For this review, take the finished solid that the model builds, in its own axes (mm). A direction names the side the tool comes from. Coordinates: 2 decimals unless noted, no trailing zeros. Write each loop counter-clockwise with the first axis right and the second up, starting at its lowest first coordinate (ties: lowest second). Pieces come first, ordered by that corner, then holes. Notation, with made-up numbers: M -40,86.5 L 7,86.5 A23 cw 7,113.5 Z; hole C 37.5,66.5 d1. An arc over 180 degrees is marked long. One line per question, with ' | ' between items.
from build123d import *

# Parameters (mm, degrees)
F0_R         = 1
F0_W         = 18
F0_H         = 10
F1_DEPTH     = 5
F0_W_2       = 21.25
F0_R_2       = 4
F2_DEPTH     = 20
F3_R         = 4
F4_DEPTH     = 25
F5_DEPTH     = 5
F6_T4_DEPTH  = 18
F7_T1_DEPTH  = 5
F7_T3_DEPTH  = 18
F7_T8_DEPTH  = 10
F7_T13_DEPTH = 10
F7_T19_DEPTH = 22.8584149398
F7_T24_DEPTH = 17.8584149398
F7_T33_DEPTH = 30.8584149398
F7_S35_R     = 4
F7_T36_DEPTH = 17
F7_T39_DEPTH = 17.8584149398
F7_S41_R     = 4
F7_T42_DEPTH = 11
F7_T48_DEPTH = 30.8584149398
F7_S50_R     = 4
F7_T51_DEPTH = 17
F7_T54_DEPTH = 17.8584149398
F7_S56_R     = 4
F7_T57_DEPTH = 11
F7_T63_DEPTH = 17.8584149398
F7_T69_DEPTH = 22.8584149398


# Not quite as in the source:
# - a fillet or chamfer that OpenCascade refuses, or shapes differently, is made with other operations: its cross-section is extruded or revolved along the edge and cut away or added
# - a feature names something its author has since deleted; it is built from what else it names


with BuildPart() as f1:
    # F0 (on Top) → F1 (new body)
    with BuildSketch(Plane.XY):
        with BuildLine():
            Line((9, 0), (4, 0))
            ThreePointArc((4, 0), (0, -4), (-4, 0))
            Line((-4, 0), (-9, 0))
            ThreePointArc((-9, 0), (0, -9), (9, 0))
        make_face()
        with Locations((-4.5, -4.5)):
            Circle(F0_R, mode=Mode.SUBTRACT)
        with Locations((4.5, -4.5)):
            Circle(F0_R, mode=Mode.SUBTRACT)
        with BuildLine():
            ThreePointArc((-4, 0), (0, 4), (4, 0))
            Line((4, 0), (9, 0))
            ThreePointArc((9, 0), (0, 9), (-9, 0))
            Line((-9, 0), (-4, 0))
        make_face()
        with BuildLine():
            ThreePointArc((-4.5, 3.5), (-5.2071067812, 5.2071067812), (-3.5, 4.5))
            ThreePointArc((-3.5, 4.5), (-3.7928932188, 3.7928932188), (-4.5, 3.5))
        make_face(mode=Mode.SUBTRACT)
        with Locations((4.5, 4.5)):
            Circle(F0_R, mode=Mode.SUBTRACT)
        with BuildLine():
            ThreePointArc((-9, 0), (0, 9), (9, 0))
            Line((9, 0), (9, 14))
            Line((9, 14), (-9, 14))
            Line((-9, 14), (-9, 0))
        make_face()
        with Locations((0, 19)):
            Rectangle(F0_W, F0_H)
    extrude(amount=F1_DEPTH)

    # F0 (on Top) → F2 (join)
    with BuildSketch(Plane.XY):
        with Locations((0, 19)):
            Rectangle(F0_W, F0_H)
        with Locations((-19.625, 19)):
            Rectangle(F0_W_2, F0_H)
        with Locations((-20.25, 19)):
            Circle(F0_R_2, mode=Mode.SUBTRACT)
        with Locations((19.625, 19)):
            Rectangle(F0_W_2, F0_H)
        with Locations((20.25, 19)):
            Circle(F0_R_2, mode=Mode.SUBTRACT)
        with Locations((20.25, 19)):
            Circle(F0_R_2)
        with Locations((-20.25, 19)):
            Circle(F0_R_2)
    extrude(amount=F2_DEPTH)

    # F3 (on Front) → F4 (cut)
    with BuildSketch(Plane.XZ):
        with Locations((-16.25, 13)):
            Circle(F3_R)
        with Locations((16.25, 13)):
            Circle(F3_R)
    extrude(amount=-F4_DEPTH, mode=Mode.SUBTRACT)

    # F0 (on Top) → F5 (join)
    with BuildSketch(Plane.XY):
        with Locations((0, 19)):
            Rectangle(F0_W, F0_H)
    extrude(amount=-F5_DEPTH)

    # F6: chamfer of 5 on 1 edges, made by hand


with BuildPart() as f6_tool2:
    # F6_s3 → F6_t4 (new body)
    with BuildSketch(Plane.YZ.offset(-9)):
        Polygon((9, 0), (14, -5), (14, 0), align=None)
    extrude(amount=F6_T4_DEPTH)

    split(bisect_by=Plane.XY.offset(-5), keep=Keep.TOP)


with BuildPart() as f1_1:
    add(f1.part)

    # F6_t1: union F6_tool2
    add(f6_tool2.part)

    # F7: chamfer of 5 on 5 edges, made by hand

    # F7_s2 → F7_t1 (join)
    with BuildSketch(Plane.XY):
        Polygon((-9, 9), (-14, 14), (-9, 14), align=None)
        Polygon((9, 9), (14, 14), (9, 14), align=None)
    extrude(amount=F7_T1_DEPTH)

    # F7_s4 → F7_t3 (join)
    with BuildSketch(Plane.YZ.offset(-9)):
        Polygon((9, 5), (14, 10), (14, 5), align=None)
    extrude(amount=F7_T3_DEPTH)


with BuildPart() as f7_tool6:
    # F7_s7 → F7_t8 (new body)
    with BuildSketch(Plane.XZ.offset(-14)):
        Polygon((9, -5), (14, 0), (9, 0), align=None)
    extrude(amount=-F7_T8_DEPTH)

    split(bisect_by=Plane.XY.offset(-5), keep=Keep.TOP)


with BuildPart() as f1_2:
    add(f1_1.part)

    # F7_t5: union F7_tool6
    add(f7_tool6.part)


with BuildPart() as f7_tool11:
    # F7_s12 → F7_t13 (new body)
    with BuildSketch(Plane.XZ.offset(-24)):
        Polygon((-9, -5), (-14, 0), (-9, 0), align=None)
    extrude(amount=F7_T13_DEPTH)

    split(bisect_by=Plane.XY.offset(-5), keep=Keep.TOP)


with BuildPart() as f1_3:
    add(f1_2.part)

    # F7_t10: union F7_tool11
    add(f7_tool11.part)


with BuildPart() as f7_tool17:
    # F7_s18 → F7_t19 (new body)
    with BuildSketch(Plane.XZ.offset(-24)):
        Polygon((-9, -5), (-14, 0), (-9, 0), align=None)
    extrude(amount=F7_T19_DEPTH)

    split(bisect_by=Plane(origin=(0, 4.5, 4.5), x_dir=(1, 0, 0), z_dir=(0, 0.7071067812, 0.7071067812)), keep=Keep.TOP)

    split(bisect_by=Plane.XZ.offset(-14), keep=Keep.TOP)


with BuildPart() as f7_tool22:
    # F7_s23 → F7_t24 (new body)
    with BuildSketch(Plane.XY.offset(-12.8584149398)):
        Polygon((-9, 9), (-14, 14), (-9, 14), align=None)
    extrude(amount=F7_T24_DEPTH)

    split(bisect_by=Plane.XY, keep=Keep.BOTTOM)

    split(bisect_by=Plane(origin=(0, 4.5, 4.5), x_dir=(1, 0, 0), z_dir=(0, 0.7071067812, 0.7071067812)), keep=Keep.TOP)

    split(bisect_by=Plane.XY.offset(-5), keep=Keep.TOP)


with BuildPart() as f7_tool17_1:
    add(f7_tool17.part)

    # F7_t28: intersect F7_tool22
    add(f7_tool22.part, mode=Mode.INTERSECT)


with BuildPart() as f1_4:
    add(f1_3.part)

    # F7_t15: union F7_tool17
    add(f7_tool17_1.part)


with BuildPart() as f7_tool31:
    # F7_s32 → F7_t33 (new body)
    with BuildSketch(Plane.YZ.offset(9)):
        Polygon((9, 5), (14, 10), (14, 5), align=None)
    extrude(amount=-F7_T33_DEPTH)

    split(bisect_by=Plane.YZ.offset(-9), keep=Keep.BOTTOM)

    # F7_s35 → F7_t36 (cut, symmetric)
    with BuildSketch(Plane.XZ.offset(-11.5)):
        with Locations((-16.25, 13)):
            Circle(F7_S35_R)
    extrude(amount=F7_T36_DEPTH, both=True, mode=Mode.SUBTRACT)


with BuildPart() as f7_tool37:
    # F7_s38 → F7_t39 (new body)
    with BuildSketch(Plane.XY):
        Polygon((-9, 9), (-14, 14), (-9, 14), align=None)
    extrude(amount=F7_T39_DEPTH)

    split(bisect_by=Plane.XY.offset(5), keep=Keep.TOP)

    # F7_s41 → F7_t42 (cut, symmetric)
    with BuildSketch(Plane.XZ.offset(-11.5)):
        with Locations((-16.25, 13)):
            Circle(F7_S41_R)
    extrude(amount=F7_T42_DEPTH, both=True, mode=Mode.SUBTRACT)


with BuildPart() as f7_tool31_1:
    add(f7_tool31.part)

    # F7_t43: intersect F7_tool37
    add(f7_tool37.part, mode=Mode.INTERSECT)


with BuildPart() as f1_5:
    add(f1_4.part)

    # F7_t29: union F7_tool31
    add(f7_tool31_1.part)


with BuildPart() as f7_tool46:
    # F7_s47 → F7_t48 (new body)
    with BuildSketch(Plane.YZ.offset(21.8584149398)):
        Polygon((9, 5), (14, 10), (14, 5), align=None)
    extrude(amount=-F7_T48_DEPTH)

    split(bisect_by=Plane.YZ.offset(9), keep=Keep.TOP)

    # F7_s50 → F7_t51 (cut, symmetric)
    with BuildSketch(Plane.XZ.offset(-11.5)):
        with Locations((16.25, 13)):
            Circle(F7_S50_R)
    extrude(amount=F7_T51_DEPTH, both=True, mode=Mode.SUBTRACT)


with BuildPart() as f7_tool52:
    # F7_s53 → F7_t54 (new body)
    with BuildSketch(Plane.XY.offset(17.8584149398)):
        Polygon((9, 9), (14, 14), (9, 14), align=None)
    extrude(amount=-F7_T54_DEPTH)

    split(bisect_by=Plane.XY.offset(5), keep=Keep.TOP)

    # F7_s56 → F7_t57 (cut, symmetric)
    with BuildSketch(Plane.XZ.offset(-11.5)):
        with Locations((16.25, 13)):
            Circle(F7_S56_R)
    extrude(amount=F7_T57_DEPTH, both=True, mode=Mode.SUBTRACT)


with BuildPart() as f7_tool46_1:
    add(f7_tool46.part)

    # F7_t58: intersect F7_tool52
    add(f7_tool52.part, mode=Mode.INTERSECT)


with BuildPart() as f1_6:
    add(f1_5.part)

    # F7_t44: union F7_tool46
    add(f7_tool46_1.part)


with BuildPart() as f7_tool61:
    # F7_s62 → F7_t63 (new body)
    with BuildSketch(Plane.XY.offset(5)):
        Polygon((9, 9), (14, 14), (9, 14), align=None)
    extrude(amount=-F7_T63_DEPTH)

    split(bisect_by=Plane.XY, keep=Keep.BOTTOM)

    split(bisect_by=Plane(origin=(0, 4.5, 4.5), x_dir=(1, 0, 0), z_dir=(0, 0.7071067812, 0.7071067812)), keep=Keep.TOP)

    split(bisect_by=Plane.XY.offset(-5), keep=Keep.TOP)


with BuildPart() as f7_tool67:
    # F7_s68 → F7_t69 (new body)
    with BuildSketch(Plane.XZ.offset(-1.1415850602)):
        Polygon((9, -5), (14, 0), (9, 0), align=None)
    extrude(amount=-F7_T69_DEPTH)

    split(bisect_by=Plane(origin=(0, 4.5, 4.5), x_dir=(1, 0, 0), z_dir=(0, 0.7071067812, 0.7071067812)), keep=Keep.TOP)

    split(bisect_by=Plane.XZ.offset(-14), keep=Keep.TOP)


with BuildPart() as f7_tool61_1:
    add(f7_tool61.part)

    # F7_t72: intersect F7_tool67
    add(f7_tool67.part, mode=Mode.INTERSECT)


with BuildPart() as f1_7:
    add(f1_6.part)

    # F7_t59: union F7_tool61
    add(f7_tool61_1.part)


solid = f1_7.part
1. Draft analysis for pull direction Y (two halves, no side actions). For faces 6 (the cylindrical face through (0.867, -3.905, 2.465)), 7 (the flat face through (11, 11, 4)), 8 (the flat face through (0, 19, -5)), state which applies: pulls with the +Y half, pulls with the -Y half, needs draft (parallel to the pull), parting line crosses it, or undercut.
Computed values:
face 6: undercut | face 7: pulls with the -Y half | face 8: needs draft
2. Take a section at A-A on x = 0. State the section outline as (y, z) points, plus the area to 3 significant figures.
Computed values:
outline: M -9,0 L -4,0 L -4,5 L -9,5 Z; M 4,0 L 9,0 L 14,-5 L 24,-5 L 24,20 L 14,20 L 14,10 L 9,5 L 4,5 Z | area: 350 mm2
3. For line 1 along X through (y, z) = (20.5, 13); line 2 along Z through (x, y) = (16.25, 22); line 3 along Y through (x, z) = (-4.5, 4), list the stretches that pass through material, from the lowest coordinate up.
Computed values:
line 1: x = -30.25 to -20.25, -12.25 to 12.25, 20.25 to 30.25 | line 2: z = 0 to 9, 17 to 20 | line 3: y = -7.79 to -5.5, -3.5 to 3.5, 5.5 to 24
4. Clearance check with flat-ended pins moving along their axes: P1, Ø2.5, axis at x = -4.5, y = -4.5, coming from the -Z side; P2, Ø2.5, axis at y = 3.5, z = 2.5, coming from the +X side; P3, Ø3, axis at x = 4.5, y = 4.5, coming from the +Z side; P4, Ø9, axis at x = 16.25, z = 13, coming from the +Y side. State where each tip first meets the part, or that it passes through.
Computed values:
P1: stops at z = 0 | P2: stops at x = 9 | P3: stops at z = 5 | P4: stops at y = 24
5. Machinability: for faces 1 (the flat face through (-2, 4, 5)), 2 (the flat face through (0, 14, 12)), 3 (the flat face through (22, 19, 0)), 4 (the flat face through (-22, 19, 0)), 5 (the flat face through (-9, 4, 3)), which of the approach directions +Z, -Z, +X, -X, +Y, -Y give a long, thin tool a straight path to every point of the face, cutting with its end or side? Answer none if there is none.
Computed values:
face 1: +Z, +X, -X, -Y | face 2: +Z, -Y | face 3: -Z, +X, +Y, -Y | face 4: -Z, -X, +Y, -Y | face 5: +Z, -Z, -X, -Y
6. Take a section at B-B on y = 16. State the section outline as (x, z) points.
Computed values:
outline: M -30.25,0 L -14,0 L -9,-5 L 9,-5 L 14,0 L 30.25,0 L 30.25,20 L -30.25,20 Z; hole C -16.25,13 d8; hole C 16.25,13 d8
7. Take a section at D-D on y = 2. State the section outline as (x, z) points, plus the area to 3 significant figures.
Computed values:
outline: M -9,0 L -3.46,0 L -3.46,5 L -9,5 Z; M 3.46,0 L 9,0 L 9,5 L 3.46,5 Z | area: 55.4 mm2
8. Take a section at C-C on z = 13. State the section outline as (x, y) points, plus the area to 3 significant figures.
Computed values:
outline: M -30.25,14 L -20.25,14 L -20.25,24 L -30.25,24 Z; M -12.25,14 L 12.25,14 L 12.25,24 L -12.25,24 Z; M 20.25,14 L 30.25,14 L 30.25,24 L 20.25,24 Z | area: 445 mm2
